from build123d import *

# Parameters (mm, degrees)
F0_W                 = 10
F0_H                 = 10
F1_DEPTH             = 10
F4_D                 = 3
F4_CSINK_D           = 9
F4_CSINK_ANGLE       = 82
F4_ON_F2_D           = 3
F4_ON_F2_CSINK_D     = 9
F4_ON_F2_CSINK_ANGLE = 82
F5_T1_DEPTH          = 15.1433659759


# Not quite as in the source:
# - a fillet or chamfer that OpenCascade refuses, or shapes differently, is made with other operations: its cross-section is extruded or revolved along the edge and cut away or added


with BuildPart() as f1:
    # F0 (on Top) → F1 (new body)
    with BuildSketch(Plane.XY):
        with BuildLine():
            ThreePointArc((27.5680975042, -33), (-18.2149911792, -38.9514325326), (-43, 0))
            Line((-43, 0), (-43, 45))
            Line((-43, 45), (-53, 45))
            Line((-53, 45), (-53, 35))
            Line((-53, 35), (-53, 0))
            ThreePointArc((-53, 0), (-24.154244567, -47.1759734335), (30.9838667697, -43))
            Line((30.9838667697, -43), (36.9838667697, -53))
            Line((36.9838667697, -53), (46.9838667697, -53))
            Line((46.9838667697, -53), (46.9838667697, -43))
            Line((46.9838667697, -43), (46.9838667697, -33))
            Line((46.9838667697, -33), (27.5680975042, -33))
        make_face()
        with Locations((-58, 40)):
            Rectangle(F0_W, F0_H)
    extrude(amount=F1_DEPTH)

    # F4 (through all)
    with Locations(Plane(origin=(3.8116667424, 2.2870000454, 0), x_dir=(0.5144957554, -0.8574929257, 0), z_dir=(-0.8574929257, -0.5144957554, 0))):
        with Locations((58.6442156402, 5)):
            CounterSinkHole(F4_D / 2, F4_CSINK_D / 2, counter_sink_angle=F4_CSINK_ANGLE)

    # F4 on F2 (through all)
    with Locations(Plane.XZ.offset(-35)):
        with Locations((-58, 5)):
            CounterSinkHole(F4_ON_F2_D / 2, F4_ON_F2_CSINK_D / 2, counter_sink_angle=F4_ON_F2_CSINK_ANGLE)

    # F5: chamfer of 1 on 1 edges, made by hand

    # F5_s2 → F5_t1 (cut)
    with BuildSketch(Plane.XY.offset(-2.571682988)):
        Polygon((-63, 36), (-62, 35), (-63, 35), align=None)
    extrude(amount=F5_T1_DEPTH, mode=Mode.SUBTRACT)


solid = f1.part
For this review, take the finished solid that the model builds, in its own axes (mm). A direction names the side the tool comes from. Round coordinates to 2 decimals unless told otherwise and drop trailing zeros. Order: outer loops, then holes, each group sorted by start corner. A loop starts at its lowest first (then second) coordinate and runs counter-clockwise, first axis right, second up. Notation, with made-up numbers: (33.5, 64.5) -> (62.5, 64.5) arc R17 ccw to (62.5, 91.5) -> close; hole circle Ø9 at (26, 33). An arc over 180 degrees is marked (long way). Write item = value, one per line. Start each with the question number.
1) To check wall thickness, follow line 1 (X direction, y = 42.5, z = 5); line 2 (Z direction, x = -58, y = 41); line 3 (Y direction, x = 31, z = 4.5). State the ranges of each line that lie inside material, in increasing order. Write a range as from..to.
2) Take a section at A-A on x = -58. State the section outline as (y, z) points.
3) Tool access review of faces 1 (the face through (33.275, -46.819, 0.486)), 2 (the face through (36.017, -45.007, 4.37)), 3 (the face through (-53.2, 35, 5)), 4 (the face through (-56.356, 38.284, 5.072)), 5 (the face through (-43, 22, 5)): name each direction out of +Z, -Z, +X, -X, +Y, -Y from which nothing blocks a thin tool from reaching the whole face with its end or side.
4) Take a section at B-B on z = 5. State the section outline as (x, y) points.
5) Take a section at C-C on y = 3.5. State the section outline as (x, z) points, plus the area to 3 significant figures.
6) The part is to be moulded in two halves that separate along X. For faces 6 (the face through (-53, 18, 5)), 7 (the face through (37, -33, 5)), 8 (the face through (41.712, -41.747, 4.425)), 9 (the face through (46.984, -43, 5)), say which applies: +X half, -X half, draft (parallel to the pull), parting line (faces both ways), or undercut.
7) Insertion check: pin 1 (1 mm diameter, centred on y = -24.5, z = 3, fed in from +X); pin 2 (3 mm diameter, centred on x = 34.5, z = 3, fed in from +Y); pin 3 (4.5 mm diameter, centred on x = -56.5, z = 7.5, fed in from -Y). Each pin has a flat end and moves straight along its axis. Give the tip position at first contact, or say it passes through.
8) Take a section at D-D on x = -12. State the section outline as (y, z) points, plus the area to 3 significant figures.
Verdict:
q1.line_1 = -63..-59.5, -56.5..-43
q1.line_2 = 0..3.5, 6.5..10
q1.line_3 = -43.03..-33
q2.outline = (35, 0) -> (45, 0) -> (45, 3.5) -> (38.45, 3.5) -> (35, 0.5) -> close; (35, 9.5) -> (38.45, 6.5) -> (45, 6.5) -> (45, 10) -> (35, 10) -> close
q3.face_1 = +Z, -Z, -Y
q3.face_2 = none
q3.face_3 = +Z, -Z, -X, -Y
q3.face_4 = -Y
q3.face_5 = +Z, -Z, +X, +Y
q4.outline = (-63, 36) -> (-62.27, 35.27) -> (-59.5, 38.45) -> (-59.5, 45) -> (-63, 45) -> close; (-56.5, 38.45) -> (-53.5, 35) -> (-53, 35) -> (-53, 0) arc R53 ccw to (30.98, -43) -> (31.67, -44.14) -> (36.17, -44.94) -> (46.98, -38.45) -> (46.98, -33) -> (27.57, -33) arc R43 cw to (-43, 0) -> (-43, 45) -> (-56.5, 45) -> close; (36.3, -51.86) -> (36.98, -53) -> (46.98, -53) -> (46.98, -41.95) -> (37.71, -47.51) -> close
q5.outline = (-53, 0) -> (-43, 0) -> (-43, 10) -> (-53, 10) -> close
q5.area = 100 mm2
q6.face_6 = -X half
q6.face_7 = draft
q6.face_8 = undercut
q6.face_9 = +X half
q7.pin_1 = -34.99
q7.pin_2 = -33
q7.pin_3 = 35
q8.outline = (-51.62, 0) -> (-41.29, 0) -> (-41.29, 10) -> (-51.62, 10) -> close
q8.area = 103 mm2
